```python
from build123d import *

# Parameters (mm, degrees)
F0_W     = 3.5
F0_H     = 61
F1_DEPTH = 2.5
F2_R     = 1
F3_ANGLE = -40
F4_W     = 59.4788547605
F4_H     = 9.7545320168
F5_DEPTH = 25


with BuildPart() as f1:
    # F0 (on Front) → F1 (new body)
    with BuildSketch(Plane.XZ):
        with Locations((-1.75, 30.5)):
            Rectangle(F0_W, F0_H)
    extrude(amount=F1_DEPTH)

    # F2
    f2_edges = [f1.edges().sort_by_distance(p)[0] for p in [
        (-3.5, -1.25, 61),
        (0, -1.25, 61),
    ]]
    fillet(f2_edges, radius=F2_R)


with BuildPart() as f1_1:
    # F3: moved
    add(f1.part.rotate(Axis((0, -1.25, 0), (0, 1, 0)), F3_ANGLE))


with BuildPart() as f5:
    # F4 (on Front) → F5 (new body)
    with BuildSketch(Plane.XZ):
        with Locations((-13.0853476003, -4.8772660084)):
            Rectangle(F4_W, F4_H)
    extrude(amount=F5_DEPTH)


with BuildPart() as f1_2:
    add(f1_1.part)

    # F6: cut F5
    add(f5.part, mode=Mode.SUBTRACT)


solid = f1_2.part
```
Geometry check sheet. Reference: the model listing, model coordinates, mm. Give positions to 0.01 mm unless a question says otherwise; leave off trailing zeros. Order: outer loops, then holes, each group sorted by start corner. A loop starts at its lowest first (then second) coordinate and runs counter-clockwise, first axis right, second up.
1. Gauge pin test, flat end, axial feed: pin 1 Ø10 at (x, z) = (-21.5, 26) entering from +Y. Record the tip position at first contact, or that the pin passes through.
2. Section check A-A, the plane y = -1.65. Enter the section's corners in (x, z), and give its area (3 significant figures).
3. Section check C-C, the plane x = -33.5. Enter the section's corners in (y, z), and give its area (3 significant figures).
4. Section check B-B, the plane z = 29.5. Enter the section's corners in (x, y), and give its area (3 significant figures).
5. Thickness scan on L1, parallel to X at y = -2, z = 35; L2, parallel to Z at x = -39, y = -1.05; L3, parallel to Z at x = -5.5, y = -0.8. Record the ranges inside material, lowest first.
Values follow:
1. pin 1: stops at y = 0
2. outline: (-41.25, 43.71) - (-4.57, 0) - (0, 0) - (-38.57, 45.96) arc R1 ccw to (-39.98, 46.09) - (-41.13, 45.12) arc R1 ccw to start
2. area: 208 mm2
3. outline: (-2.5, 34.48) - (0, 34.48) - (0, 39.92) - (-2.5, 39.92) - close
3. area: 13.6 mm2
4. outline: (-29.32, -2.5) - (-24.75, -2.5) - (-24.75, 0) - (-29.32, 0) - close
4. area: 11.4 mm2
5. L1: x = -33.94 to -29.37
5. L2: z = 41.03 to 46.26
5. L3: z = 1.11 to 6.55
